```python
from build123d import *

# Parameters (mm, degrees)
CROQUIS1_R                 = 13.5
SALIENTE_EXTRUIR1_DEPTH    = 11.5
CROQUIS3_R                 = 2
CORTAR_EXTRUIR1_DEPTH      = 34.535832747
CORTAR_EXTRUIR2_DEPTH      = 34.535832747
CORTAR_EXTRUIR2_DEPTH_BACK = 34.535832747
REDONDEO1_R                = 20
REDONDEO2_R                = 11.5
CROQUIS5_R                 = 6
CORTAR_EXTRUIR3_DEPTH      = 7
CROQUIS6_R                 = 9.5
CORTAR_EXTRUIR4_DEPTH      = 5
CROQUIS7_R                 = 1.5
CORTAR_EXTRUIR5_DEPTH      = 33.099173306


with BuildPart() as part:
    # Croquis1 → Saliente-Extruir1 (new body)
    with BuildSketch(Plane.XY):
        with BuildLine():
            Line((0.447526726, 13.492580177), (-28, 14.436137919))
            Line((-28, 14.436137919), (-28, -14.436137919))
            Line((-28, -14.436137919), (0.447526726, -13.492580177))
            ThreePointArc((0.447526726, -13.492580177), (-13.5, 0), (0.447526726, 13.492580177))
        make_face()
        Circle(CROQUIS1_R)
    extrude(amount=SALIENTE_EXTRUIR1_DEPTH)

    # Croquis3 → Cortar-Extruir1 (cut, through all)
    with BuildSketch(Plane.XY.offset(11.5)):
        with Locations((-22, 0)):
            Circle(CROQUIS3_R)
        with Locations((-19.602143532, 9.987790994)):
            Circle(CROQUIS3_R)
        with Locations((-11.490666647, 9.641814145)):
            Circle(CROQUIS3_R)
        with Locations(Location((-19.602143532, -9.987790994, 0), (0, 0, 180))):
            Circle(CROQUIS3_R)
        with Locations(Location((-11.490666647, -9.641814145, 0), (0, 0, 180))):
            Circle(CROQUIS3_R)
    extrude(amount=-CORTAR_EXTRUIR1_DEPTH, mode=Mode.SUBTRACT)

    # Croquis4 → Cortar-Extruir2 (cut, two sides: drawn at the far end of the back side and taken through both)
    with BuildSketch(Plane(origin=(0, 0, 0), x_dir=(1, 0, 0), z_dir=(0, 1, 0)).offset(-CORTAR_EXTRUIR2_DEPTH_BACK)):
        Polygon((-15, 0), (-28, -5.75), (-28, 0), align=None)
    extrude(amount=CORTAR_EXTRUIR2_DEPTH + CORTAR_EXTRUIR2_DEPTH_BACK, mode=Mode.SUBTRACT)

    # Redondeo1
    # the kernel refuses this fillet: 20 mm, written as the material it takes off along each edge
    with BuildSketch(Plane(origin=(-15, -24.56902732, 0), x_dir=(1, 0, 0), z_dir=(0, 1, 0))) as redondeo1_piece_1:
        with BuildLine():
            CenterArc((REDONDEO1_R * 0.211281561014, -REDONDEO1_R), REDONDEO1_R, 90, 23.860175191)
            Line((-REDONDEO1_R * 0.193224453764, -REDONDEO1_R * 0.0854646622417), (0, 0))
            Line((0, 0), (REDONDEO1_R * 0.211281561014, 0))
        make_face()
    extrude(amount=49.138054639, mode=Mode.SUBTRACT)

    # Redondeo2
    # the kernel refuses this fillet: 11.5 mm, written as the material it takes off along each edge
    with BuildSketch(Plane(origin=(-28, 14.436137919, -23.969400449), x_dir=(0.9994503834734472, -0.033150127824481866, 0), z_dir=(0, 0, 1))) as redondeo2_piece_1:
        with BuildLine():
            CenterArc((REDONDEO2_R * 1.03371827647, -REDONDEO2_R), REDONDEO2_R, 90, 91.899710465)
            Line((REDONDEO2_R * 0.0342678929996, -REDONDEO2_R * 1.03315012782), (0, 0))
            Line((0, 0), (REDONDEO2_R * 1.03371827647, 0))
        make_face()
    extrude(amount=65.188800897, mode=Mode.SUBTRACT)
    with BuildSketch(Plane(origin=(-28, -14.436137919, -23.969400449), x_dir=(0.999450383473447, 0.033150127824482116, 0), z_dir=(0, 0, 1))) as redondeo2_piece_2:
        with BuildLine():
            CenterArc((REDONDEO2_R * 1.03371827647, REDONDEO2_R), REDONDEO2_R, 178.100289535, 91.899710465)
            Line((REDONDEO2_R * 0.0342678929996, REDONDEO2_R * 1.03315012782), (0, 0))
            Line((0, 0), (REDONDEO2_R * 1.03371827647, 0))
        make_face()
    extrude(amount=65.188800897, mode=Mode.SUBTRACT)

    # Croquis5 → Cortar-Extruir3 (cut)
    with BuildSketch(Plane(origin=(0, 0, 0), x_dir=(-1, 0, 0), z_dir=(0, 0, -1))):
        Circle(CROQUIS5_R)
    extrude(amount=-CORTAR_EXTRUIR3_DEPTH, mode=Mode.SUBTRACT)

    # Croquis6 → Cortar-Extruir4 (cut)
    with BuildSketch(Plane(origin=(0, 0, 0), x_dir=(-1, 0, 0), z_dir=(0, 0, -1))):
        Circle(CROQUIS6_R)
    extrude(amount=-CORTAR_EXTRUIR4_DEPTH, mode=Mode.SUBTRACT)

    # Croquis7 → Cortar-Extruir5 (cut, through all)
    with BuildSketch(Plane(origin=(0, 0, 7), x_dir=(-1, 0, 0), z_dir=(0, 0, -1))):
        Circle(CROQUIS7_R)
    extrude(amount=-CORTAR_EXTRUIR5_DEPTH, mode=Mode.SUBTRACT)


solid = part.part
```
Could you check a few things on this model? Use its own coordinates, in mm. A direction names the side the tool comes from. Coordinates: 2 decimals unless noted, no trailing zeros. Loops run counter-clockwise (first coordinate to the right, second up) from the corner with the lowest first, then second, coordinate; pieces in that order, holes last. Notation, with made-up numbers: M 69.5,-5 L 96.5,-5 A27 ccw 96.5,23 Z; hole C 10,15.5 d2. An arc over 180 degrees is marked long. Put each result on its own line as item: value. Start each with the question number.
(1) Will these pins go through, and if not, where does the flat tip stop? P1, Ø9.5, axis at x = 0.5, y = -1.5, coming from the -Z side; P2, Ø6, axis at x = -23.5, z = 2.5, coming from the +Y side; P3, Ø6, axis at x = 4, z = 5.5, coming from the +Y side.
(2) Suppose I cut it at D-D on x = 0. Please give me the cut outline in (y, z), then the cut area to 3 significant figures.
(3) Suppose I cut it at B-B on z = 3.5. Please give me the cut outline in (x, y), then the cut area to 3 significant figures.
(4) Thinking about a two-plate mould opening in X: for faces 3 (the face through (-28, 0, 9)), 4 (the face through (-9.493, -9.73, 5.83)), 5 (the face through (-8, 0, 11.5)), which applies, pulls with the +X half, pulls with the -X half, needs draft (parallel to the pull), parting line crosses it, or undercut?
(5) For faces 1 (the face through (-4.38, -8.43, 2.46)), 2 (the face through (-18.015, -8.771, 6.423)), which set-ups out of +Z, -Z, +X, -X, +Y, -Y let a thin tool reach every point of the face, with its end or its side?
(6) Suppose I cut it at C-C on x = -20.5. Please give me the cut outline in (y, z).
(7) I need wall thicknesses on line 1 (X direction, y = -8.25, z = 8.25); line 2 (Y direction, x = -21, z = 5.25); line 3 (Z direction, x = -3, y = -0.5). Which ranges of each line are inside material? Lowest first, please. Write a range as from..to.
(8) Suppose I cut it at A-A on y = 0. Please give me the cut outline in (x, z), then the cut area to 3 significant figures.
Solutions:
1. P1: stops at z = 5
1. P2: stops at y = 13.33
1. P3: stops at y = 13.46
2. outline: M -13.51,0 L -9.5,0 L -9.5,5 L -6,5 L -6,7 L -1.5,7 L -1.5,11.5 L -13.51,11.5 Z; M 1.5,7 L 6,7 L 6,5 L 9.5,5 L 9.5,0 L 13.51,0 L 13.51,11.5 L 1.5,11.5 Z
2. area: 178 mm2
3. outline: M -22.91,-12.09 A11.5 ccw -16.12,-14.04 L 0.45,-13.49 A13.5 ccw 0.45,13.49 L -16.12,14.04 A11.5 ccw -22.91,12.09 L -22.91,1.78 A2 cw long -22.91,-1.78 Z; hole C -19.6,-9.99 d4; hole C -19.6,9.99 d4; hole C -11.49,-9.64 d4; hole C -11.49,9.64 d4; hole C 0,0 d19
3. area: 570 mm2
4. face 3: pulls with the -X half
4. face 4: undercut
4. face 5: needs draft
5. face 1: -Z
5. face 2: +Z, -Z
6. outline: M -13.33,2.43 L -11.77,2.43 L -11.77,11.5 L -13.33,11.5 Z; M -8.2,2.43 L -1.32,2.43 L -1.32,11.5 L -8.2,11.5 Z; M 1.32,2.43 L 8.2,2.43 L 8.2,11.5 L 1.32,11.5 Z; M 11.77,2.43 L 13.33,2.43 L 13.33,11.5 L 11.77,11.5 Z
7. line 1: x = -26.49..-20.59, -18.61..-12.93, -10.05..10.69
7. line 2: y = -13.13..-11.42, -8.56..-1.73, 1.73..8.56, 11.42..13.13
7. line 3: z = 7..11.5
8. outline: M -28,5.75 L -24,3.98 L -24,11.5 L -28,11.5 Z; M -20,2.21 L -18.86,1.71 A20 ccw -10.77,0 L -9.5,0 L -9.5,5 L -6,5 L -6,7 L -1.5,7 L -1.5,11.5 L -20,11.5 Z; M 1.5,7 L 6,7 L 6,5 L 9.5,5 L 9.5,0 L 13.5,0 L 13.5,11.5 L 1.5,11.5 Z
8. area: 273 mm2
